For this review, take the finished solid that the model builds, in its own axes (mm). Face numbers are marked on the shaded views. A direction names the side the tool comes from. Round coordinates to 2 decimals unless told otherwise and drop trailing zeros. Loops run counter-clockwise (first coordinate to the right, second up) from the corner with the lowest first, then second, coordinate; pieces in that order, holes last. Notation, with made-up numbers: (44, -3) -> (64, -3) arc R28 ccw to (64, 35) -> close; hole circle Ø5 at (8.5, 58.5). An arc over 180 degrees is marked (long way). One line per question, with ' | ' between items. Start each with the question number.
1. Consider section B-B (y = 11.5). Write out the cut boundary in (x, z), and give its area (3 significant figures).
2. Wall thickness on line 1 along X through (y, z) = (1.05, 0); line 2 along X through (y, z) = (2, 1); line 3 along Y through (x, z) = (-8, 1.5): over which ranges is each line inside the solid? List them lowest first.
3. For pin 1 Ø4 at (y, z) = (22, 19) entering from +X; pin 2 Ø2 at (x, z) = (9.5, 9.5) entering from +Y; pin 3 Ø6 at (y, z) = (22.5, 19.45) entering from -X, all flat-tipped, find the tip position at first contact; note any pin that passes through.
4. For the marked faces 1 and 2, list the 3-axis set-ups (+Z, -Z, +X, -X, +Y, -Y) from which the entire face can be reached by the end or side of a thin tool; tool diameter is ignored.
5. Consider section A-A (x = 0). Count the separate pieces of the cut face and the enclosed holes in it, and give its area (3 significant figures).
6. Draft analysis for pull direction Z (two halves, no side actions). For the marked faces 3, 4 and 5, state which applies: pulls with the +Z half, pulls with the -Z half, needs draft (parallel to the pull), parting line crosses it, or undercut.
```python
from build123d import *

# Parameters (mm, degrees)
BOSS_EXTRUDE3_DEPTH     = 1
BOSS_EXTRUDE4_DEPTH     = 19.6
CUT_EXTRUDE3_START      = -1
CUT_EXTRUDE3_DEPTH      = 38.799803657
BOSS_EXTRUDE5_DEPTH     = 30
CUT_EXTRUDE4_DEPTH      = 42.354259319
CUT_EXTRUDE4_DEPTH_BACK = 42.354259319
SKETCH9_R               = 2
BOSS_EXTRUDE6_DEPTH     = 17.6
SKETCH10_R              = 3.55
BOSS_EXTRUDE7_DEPTH     = 1
SKETCH11_R              = 1.8
CUT_EXTRUDE5_DEPTH      = 2
SKETCH12_R              = 4.5
BOSS_EXTRUDE8_DEPTH     = 2
SKETCH13_R              = 10.05
SKETCH13_R_2            = 5.1
BOSS_EXTRUDE9_DEPTH     = 2
SKETCH14_R              = 2.6
CUT_EXTRUDE6_DEPTH      = 39.097569002
FILLET2_R               = 2
FILLET3_R               = 2
FILLET4_R               = 2
FILLET5_R               = 2


# Some blends are built 0.0001 mm under size
with BuildPart() as part:
    # Sketch1 → Boss-Extrude3 (new body)
    # profile 1 of 2: a face of its own
    with BuildSketch(Plane(origin=(0, 0, 0), x_dir=(1, 0, 0), z_dir=(0, 1, 0))):
        with BuildLine():
            Line((9.8, -7.762087348), (9.8, -16.888723439))
            Line((9.8, -16.888723439), (-9.8, -16.888723439))
            Line((-9.8, -16.888723439), (-9.8, -7.762087348))
            ThreePointArc((-9.8, -7.762087348), (-9.848151778, -7.455517678), (-9.987969925, -7.178471758))
            ThreePointArc((-9.987969925, -7.178471758), (0, 12.3), (9.987969925, -7.178471758))
            ThreePointArc((9.987969925, -7.178471758), (9.848151778, -7.455517678), (9.8, -7.762087348))
        make_face()
        with BuildLine():
            ThreePointArc((8.8, -7.762087348), (8.896303556, -7.148948009), (9.17593985, -6.594856168))
            ThreePointArc((9.17593985, -6.594856168), (0, 11.3), (-9.17593985, -6.594856168))
            ThreePointArc((-9.17593985, -6.594856168), (-8.896303556, -7.148948009), (-8.8, -7.762087348))
            Line((-8.8, -7.762087348), (-8.8, -15.888723439))
            Line((-8.8, -15.888723439), (8.8, -15.888723439))
            Line((8.8, -15.888723439), (8.8, -7.762087348))
        make_face(mode=Mode.SUBTRACT)
    # profile 2 of 2: a face of its own
    with BuildSketch(Plane(origin=(0, 0, 0), x_dir=(1, 0, 0), z_dir=(0, 1, 0))):
        with BuildLine():
            Line((8.8, -7.762087348), (8.8, -15.888723439))
            Line((8.8, -15.888723439), (-8.8, -15.888723439))
            Line((-8.8, -15.888723439), (-8.8, -7.762087348))
            ThreePointArc((-8.8, -7.762087348), (-8.896303556, -7.148948009), (-9.17593985, -6.594856168))
            ThreePointArc((-9.17593985, -6.594856168), (0, 11.3), (9.17593985, -6.594856168))
            ThreePointArc((9.17593985, -6.594856168), (8.896303556, -7.148948009), (8.8, -7.762087348))
        make_face()
    extrude(amount=BOSS_EXTRUDE3_DEPTH)

    # Sketch2 → Boss-Extrude4 (add)
    with BuildSketch(Plane.ZY.offset(9.8)):
        with BuildLine():
            Line((16.888723439, 0), (24.17200628, 20.851200177))
            ThreePointArc((24.17200628, 20.851200177), (22.22483795, 26.660481625), (16.113586017, 26.22251443))
            Line((16.113586017, 26.22251443), (7.762087348, 18.73346191))
            Line((7.762087348, 18.73346191), (7.762087348, 0))
            Line((7.762087348, 0), (16.888723439, 0))
        make_face()
    extrude(amount=-BOSS_EXTRUDE4_DEPTH)

    # Sketch4 → Cut-Extrude3 (cut, through all)
    with BuildSketch(Plane.XZ.offset(CUT_EXTRUDE3_START)):
        Polygon((8.8, 7.762087348), (8.8, 15.888723439), (8.8, 29.007134954), (-8.8, 29.007134954), (-8.8, 15.888723439), (-8.8, 7.762087348), align=None)
    extrude(amount=-CUT_EXTRUDE3_DEPTH, mode=Mode.SUBTRACT)

    # Sketch5 → Boss-Extrude5 (add)
    with BuildSketch(Plane(origin=(0, 1, 0), x_dir=(1, 0, 0), z_dir=(0, 1, 0))):
        with BuildLine():
            Line((-8.8, -7.762087348), (-9.8, -7.762087348))
            ThreePointArc((-9.8, -7.762087348), (-9.848151778, -7.455517678), (-9.987969925, -7.178471758))
            ThreePointArc((-9.987969925, -7.178471758), (0, 12.3), (9.987969925, -7.178471758))
            ThreePointArc((9.987969925, -7.178471758), (9.848151778, -7.455517678), (9.8, -7.762087348))
            Line((9.8, -7.762087348), (8.8, -7.762087348))
            ThreePointArc((8.8, -7.762087348), (8.896303556, -7.148948009), (9.17593985, -6.594856168))
            ThreePointArc((9.17593985, -6.594856168), (0, 11.3), (-9.17593985, -6.594856168))
            ThreePointArc((-9.17593985, -6.594856168), (-8.896303556, -7.148948009), (-8.8, -7.762087348))
        make_face()
    extrude(amount=BOSS_EXTRUDE5_DEPTH)

    # Sketch7 → Cut-Extrude4 (cut, two sides: drawn at the far end of the back side and taken through both)
    with BuildSketch(Plane(origin=(0, 0, 0), x_dir=(0, 0, -1), z_dir=(1, 0, 0)).offset(-CUT_EXTRUDE4_DEPTH_BACK)):
        Polygon((15.143665649, 54.023758671), (-16.113586017, 54.023758671), (-16.113586017, 26.22251443), (-7.762087348, 18.73346191), (6.433392437, 6.003927025), (15.143665649, 6.003927025), align=None)
    extrude(amount=CUT_EXTRUDE4_DEPTH + CUT_EXTRUDE4_DEPTH_BACK, mode=Mode.SUBTRACT)

    # Sketch9 → Boss-Extrude6 (add)
    with BuildSketch(Plane(origin=(-8.8, 0, 0), x_dir=(0, 0, -1), z_dir=(1, 0, 0))):
        with Locations(Location((-19.451682229, 22.5, 0), (0, 0, 180))):
            Circle(SKETCH9_R)
    extrude(amount=BOSS_EXTRUDE6_DEPTH)

    # Sketch10 → Boss-Extrude7 (add)
    with BuildSketch(Plane.ZY.offset(9.8)):
        with Locations(Location((19.451682229, 22.5, 0), (0, 0, 180))):
            Circle(SKETCH10_R)
    extrude(amount=BOSS_EXTRUDE7_DEPTH)

    # Sketch11 → Cut-Extrude5 (cut)
    with BuildSketch(Plane.ZY.offset(10.8)):
        with Locations((19.451682229, 22.5)):
            Circle(SKETCH11_R)
    extrude(amount=-CUT_EXTRUDE5_DEPTH, mode=Mode.SUBTRACT)

    # Sketch12 → Boss-Extrude8 (add)
    with BuildSketch(Plane(origin=(9.8, 0, 0), x_dir=(0, 0, -1), z_dir=(1, 0, 0))):
        with Locations((-19.451682229, 22.5)):
            Circle(SKETCH12_R)
    extrude(amount=BOSS_EXTRUDE8_DEPTH)

    # Sketch13 → Boss-Extrude9 (add)
    with BuildSketch(Plane(origin=(0, 1, 0), x_dir=(1, 0, 0), z_dir=(0, 1, 0))):
        with Locations(Location((0, 0, 0), (0, 0, 270))):
            Circle(SKETCH13_R)
        with Locations(Location((0, 0, 0), (0, 0, 270))):
            Circle(SKETCH13_R_2, mode=Mode.SUBTRACT)
    extrude(amount=BOSS_EXTRUDE9_DEPTH)

    # Sketch14 → Cut-Extrude6 (cut, through all)
    with BuildSketch(Plane(origin=(0, 1, 0), x_dir=(1, 0, 0), z_dir=(0, 1, 0))):
        with Locations(Location((0, 0, 0), (0, 0, 270))):
            Circle(SKETCH14_R)
    extrude(amount=-CUT_EXTRUDE6_DEPTH, mode=Mode.SUBTRACT)

    # Fillet2
    fillet2_edges = [part.edges().sort_by_distance(p)[0] for p in [
        (0, 3, -5.1),
    ]]
    fillet(fillet2_edges, radius=FILLET2_R - 0.0001)  # a hair under: the kernel refuses the full size

    # Fillet3
    fillet3_edges = [part.edges().sort_by_distance(p)[0] for p in [
        (0, 3, -10.05),
    ]]
    fillet(fillet3_edges, radius=FILLET3_R - 0.0001)  # a hair under: the kernel refuses the full size

    # Fillet4
    # the kernel refuses this fillet: 2 mm, written as the material it takes off along each edge
    with BuildSketch(Plane(origin=(-10.8, 22.5, 19.451682229), x_dir=(0, 0, -1), z_dir=(0, 1, 0))) as fillet4_piece_1:
        with BuildLine():
            CenterArc((1.817949192, -2), FILLET4_R, 30, 60)
            Line((1.817949192, 0), (1.817949192, 0.04))
            Line((1.817949192, 0.04), (3.55, 0.04))
            Line((3.55, 0.04), (3.59, 0))
            ThreePointArc((3.59, 0), (3.59, -0.5), (3.584641016, -0.98))
            Line((3.584641016, -0.98), (3.55, -1))
        make_face()
    revolve(axis=Axis((-10.8, 22.5, 19.451682229), (-1, 0, 0)), mode=Mode.SUBTRACT)

    # Fillet5
    fillet5_edges = [part.edges().sort_by_distance(p)[0] for p in [
        (11.8, 22.5, 23.951682229),
    ]]
    fillet(fillet5_edges, radius=FILLET5_R - 0.0001)  # a hair under: the kernel refuses the full size


solid = part.part
```
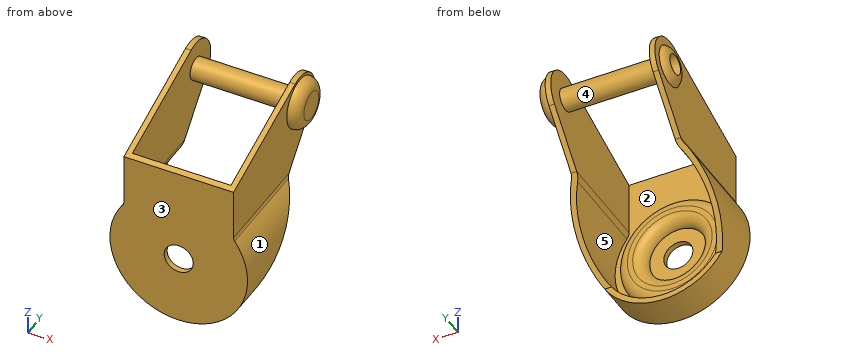
Answer block:
1) outline: (-12.3, -0.3) -> (-11.3, -0.3) arc R11.3 cw to (-9.18, 6.59) arc R2 ccw to (-8.8, 7.76) -> (-8.8, 20.91) -> (-9.8, 20.91) -> (-9.8, 7.76) arc R1 cw to (-9.99, 7.18) arc R12.3 ccw to start; (8.8, 7.76) arc R2 ccw to (9.18, 6.59) arc R11.3 cw to (11.3, -0.3) -> (12.3, -0.3) arc R12.3 ccw to (9.99, 7.18) arc R1 cw to (9.8, 7.76) -> (9.8, 20.91) -> (8.8, 20.91) -> close | area: 43.5 mm2
2) line 1: x = -12.3 to -11.3, -10.05 to -5.1, 5.1 to 10.05, 11.3 to 12.3 | line 2: x = -12.26 to -11.26, -9.73 to -5.27, 5.27 to 9.73, 11.26 to 12.26 | line 3: y = 0 to 3
3) pin 1: stops at x = 11.8 | pin 2: stops at y = 21.19 | pin 3: stops at x = -10.8
4) face 1: +Y, -Y | face 2: +Y
5) separate pieces: 3 | enclosed holes: 0 | area: 58.1 mm2
6) face 3: needs draft | face 4: parting line crosses it | face 5: undercut
